from build123d import *

# Parameters (mm, degrees)
BOSS_EXTRUDE1_DEPTH = 15
SKETCH3_OUTSIDE_W   = 28.926
SKETCH3_OUTSIDE_H   = 31.914
SKETCH3_OUTSIDE_R   = 7
CUT_EXTRUDE1_DEPTH  = 8
SKETCH4_R           = 5.5
CUT_EXTRUDE2_DEPTH  = 4
CUT_EXTRUDE3_DEPTH  = 4
SKETCH6_R           = 3
CUT_EXTRUDE4_DEPTH  = 8


with BuildPart() as part:
    # Sketch1 → Boss-Extrude1 (new body)
    with BuildSketch(Plane(origin=(0, 0, 0), x_dir=(1, 0, 0), z_dir=(0, 1, 0))):
        Polygon((9.946043617, 5.865965368), (-0.107053218, 11.546509124), (-10.053096835, 5.680543756), (-9.946043617, -5.865965368), (0.107053218, -11.546509124), (10.053096835, -5.680543756), align=None)
    extrude(amount=BOSS_EXTRUDE1_DEPTH)

    # Sketch3 outside → Cut-Extrude1 (cut)
    with BuildSketch(Plane(origin=(0, 15, 0), x_dir=(1, 0, 0), z_dir=(0, 1, 0))):
        Rectangle(SKETCH3_OUTSIDE_W, SKETCH3_OUTSIDE_H)
        Circle(SKETCH3_OUTSIDE_R, mode=Mode.SUBTRACT)
    extrude(amount=-CUT_EXTRUDE1_DEPTH, mode=Mode.SUBTRACT)

    # Sketch4 → Cut-Extrude2 (cut)
    with BuildSketch(Plane(origin=(0, 15, 0), x_dir=(1, 0, 0), z_dir=(0, 1, 0))):
        Circle(SKETCH4_R)
    extrude(amount=-CUT_EXTRUDE2_DEPTH, mode=Mode.SUBTRACT)

    # Sketch5 → Cut-Extrude3 (cut)
    with BuildSketch(Plane(origin=(0, 11, 0), x_dir=(1, 0, 0), z_dir=(0, 1, 0))):
        Polygon((-4.071504218, 2.300620221), (-4.028147665, -2.375715974), (0.043356553, -4.676336195), (4.071504218, -2.300620221), (4.028147665, 2.375715974), (-0.043356553, 4.676336195), align=None)
    extrude(amount=-CUT_EXTRUDE3_DEPTH, mode=Mode.SUBTRACT)

    # Sketch6 → Cut-Extrude4 (cut, through all)
    with BuildSketch(Plane(origin=(0, 7, 0), x_dir=(1, 0, 0), z_dir=(0, 1, 0))):
        Circle(SKETCH6_R)
    extrude(amount=-CUT_EXTRUDE4_DEPTH, mode=Mode.SUBTRACT)


solid = part.part
For this review, take the finished solid that the model builds, in its own axes (mm). A direction names the side the tool comes from. Round coordinates to 2 decimals unless told otherwise and drop trailing zeros. Write each loop counter-clockwise with the first axis right and the second up, starting at its lowest first coordinate (ties: lowest second). Pieces come first, ordered by that corner, then holes. Notation, with made-up numbers: (20, 10) - (69, 10) arc R24 ccw to (69, 21) - close; hole circle Ø6 at (-21, -37). An arc over 180 degrees is marked (long way). Use a Markdown table: item, result.
Q1. We need section B-B (x = -1.25). Give the boundary of the cut face in (y, z).
Derived:
| item | result |
|---|---|
| outline | (0, -10.87) - (7, -10.87) - (7, -6.89) - (15, -6.89) - (15, -5.36) - (11, -5.36) - (11, -3.96) - (7, -3.96) - (7, -2.73) - (0, -2.73) - close; (0, 2.73) - (7, 2.73) - (7, 3.95) - (11, 3.95) - (11, 5.36) - (15, 5.36) - (15, 6.89) - (7, 6.89) - (7, 10.78) - (0, 10.78) - close |
Q2. Clearance check with flat-ended pins moving along their axes: pin 1 (1 mm diameter, centred on x = 1.5, y = 11, fed in from -Z); pin 2 (1.5 mm diameter, centred on y = 8.5, z = 0, fed in from -X); pin 3 (1.5 mm diameter, centred on x = 6, y = 5, fed in from -Z); pin 4 (3.5 mm diameter, centred on x = 0, z = 0, fed in from +Y). State where each tip first meets the part, or that it passes through.
Derived:
| item | result |
|---|---|
| pin 1 | stops at z = -6.93 |
| pin 2 | stops at x = -7 |
| pin 3 | stops at z = -8.52 |
| pin 4 | passes through |
Q3. We need section D-D (x = -3.5). Give the boundary of the cut face in (y, z).
Derived:
| item | result |
|---|---|
| outline | (0, -9.55) - (7, -9.55) - (7, -6.06) - (15, -6.06) - (15, -4.24) - (11, -4.24) - (11, -2.64) - (7, -2.64) - (7, 2.67) - (11, 2.67) - (11, 4.24) - (15, 4.24) - (15, 6.06) - (7, 6.06) - (7, 9.51) - (0, 9.51) - close |
Q4. Machinability: for faces 5 (the flat face through (-2.4, 0, 2.4)), 6 (the flat face through (-2.029, 9.028, -3.505)), which of the approach directions +Z, -Z, +X, -X, +Y, -Y give a long, thin tool a straight path to every point of the face, cutting with its end or side? Answer none if there is none.
Derived:
| item | result |
|---|---|
| face 5 | +Z, -Z, +X, -X, -Y |
| face 6 | +Y |
Q5. The part is to be moulded in two halves that separate along X. For faces 1 (the flat face through (-4.99, 3.451, 8.666)), 2 (the cylindrical face through (6.466, 11.056, 2.681)), 3 (the flat face through (1, 7, 3)), 4 (the flat face through (-2.02, 9.03, 3.51)), say which applies: pulls with the +X half, pulls with the -X half, needs draft (parallel to the pull), parting line crosses it, or undercut.
Derived:
| item | result |
|---|---|
| face 1 | pulls with the -X half |
| face 2 | parting line crosses it |
| face 3 | undercut |
| face 4 | undercut |
Q6. We need section C-C (z = 0). Give the boundary of the cut face in (x, y), plus the area to 3 significant figures.
Derived:
| item | result |
|---|---|
| outline | (-10, 0) - (-3, 0) - (-3, 7) - (-4.05, 7) - (-4.05, 11) - (-5.5, 11) - (-5.5, 15) - (-7, 15) - (-7, 7) - (-10, 7) - close; (3, 0) - (10, 0) - (10, 7) - (7, 7) - (7, 15) - (5.5, 15) - (5.5, 11) - (4.05, 11) - (4.05, 7) - (3, 7) - close |
| area | 134 mm2 |
Q7. We need section A-A (y = 5). Give the boundary of the cut face in (x, z).
Derived:
| item | result |
|---|---|
| outline | (-10.05, -5.68) - (-0.11, -11.55) - (9.95, -5.87) - (10.05, 5.68) - (0.11, 11.55) - (-9.95, 5.87) - close; hole circle Ø6 at (0, 0) |
Q8. Wall thickness on line 1 along X through (y, z) = (12.5, 0); line 2 along Y through (x, z) = (-4.5, -1): over which ranges is each line inside the solid? List them lowest first.
Derived:
| item | result |
|---|---|
| line 1 | x = -7 to -5.5, 5.5 to 7 |
| line 2 | y = 0 to 11 |
